Autodesk Inventor part; units mm, degrees
ref_plane "YZ Plane" through (0, 0, 0) normal (1, 0, 0) x (0, 1, 0)
ref_plane "XZ Plane" through (0, 0, 0) normal (0, 1, 0) x (-1, 0, 0)
ref_plane "XY Plane" through (0, 0, 0) normal (0, 0, 1) x (1, 0, 0)
sketch "Sketch2" plane through (0, 0, 0) normal (0, 1, 0) x (-1, 0, 0)
  circle A0 centre (0, 0) radius 10 construction
  circle A1 centre (0, 0) radius 9.9
  circle A2 centre (0, 0) radius 5 construction
  circle A3 centre (0, 0) radius 7 construction
  point P0 (0, 7)
  dimension "d8" = 14
  dimension "d5" = 20
  dimension "d6" = 0.1
  dimension "d7" = 10
extrude "Extrusion1" add sketch "Sketch2" along normal blind 3
sketch "Sketch3" plane through (0, 3, 0) normal (0, 1, 0) x (1, 0, 0)
  circle A0 centre (0, 0) radius 6.5 construction
  circle A1 centre (-6.5, 0) radius 0.75
  circle A2 centre (0, 0) radius 4
  circle A3 centre (0, 0) radius 8.5 construction
  circle A4 centre (0, -6.5) radius 2
  circle A5 centre (0, 6.5) radius 2
  circle A6 centre (-6.256, 1.7644) radius 0.75
  circle A7 centre (-5.5422, 3.3962) radius 0.75
  circle A8 centre (-4.4122, 4.7731) radius 0.75
  circle A9 centre (-2.9509, 5.7915) radius 0.75
  circle A10 centre (-6.256, -1.7644) radius 0.75
  circle A11 centre (-5.5422, -3.3962) radius 0.75
  circle A12 centre (-4.4122, -4.7731) radius 0.75
  circle A13 centre (-2.9509, -5.7915) radius 0.75
  circle A14 centre (-8.5, 0) radius 0.75
  circle A15 centre (-8.1604, -2.3785) radius 0.75
  circle A16 centre (-7.1688, -4.567) radius 0.75
  circle A17 centre (-5.6044, -6.3906) radius 0.75
  circle A18 centre (-3.5923, -7.7036) radius 0.75
  circle A19 centre (-8.1604, 2.3785) radius 0.75
  circle A20 centre (-7.1688, 4.567) radius 0.75
  circle A21 centre (-5.6044, 6.3906) radius 0.75
  circle A22 centre (-3.5923, 7.7036) radius 0.75
  circle A23 centre (0, 0) radius 9.9
  line L0 (0, -9.9) -> (0, 9.9) construction
  circle A24 centre (6.5, 0) radius 0.75
  circle A25 centre (6.256, 1.7644) radius 0.75
  circle A26 centre (5.5422, 3.3962) radius 0.75
  circle A27 centre (4.4122, 4.7731) radius 0.75
  circle A28 centre (2.9509, 5.7915) radius 0.75
  circle A29 centre (6.256, -1.7644) radius 0.75
  circle A30 centre (5.5422, -3.3962) radius 0.75
  circle A31 centre (4.4122, -4.7731) radius 0.75
  circle A32 centre (2.9509, -5.7915) radius 0.75
  arc A33 (3.5923, -7.7036) -> (8.5, 0) centre (0, 0) ccw construction
  circle A34 centre (3.5923, -7.7036) radius 0.35
  circle A35 centre (6.6057, -5.3492) radius 0.35
  circle A36 centre (8.2821, -1.9121) radius 0.35
  circle A37 centre (8.2821, 1.9121) radius 0.35
  circle A38 centre (6.6057, 5.3492) radius 0.35
  circle A39 centre (3.5923, 7.7036) radius 0.35
  dimension "d14" = 13
  dimension "d15" = 1.5
  dimension "d16" = 8
  dimension "d17" = 17
  dimension "d18" = 4
  dimension "d19" = 4
  dimension "d22" = 63
  dimension "d26" = 63
  dimension "d28" = 1.5
  dimension "d31" = 65
  dimension "d35" = 65
  dimension "d37" = 0.7
  dimension "d40" = 130
extrude "Extrusion2" cut sketch "Sketch3" against normal blind 3 contours A1 | A2 | A4 | A5 | A6 | A7 | A8 | A9 | A10 | A11 | A12 | A13 | A14 | A15 | A16 | A17 | A18 | A19 | A20 | A21 | A22 | A24 | A25 | A26 | A27 | A28 | A29 | A30 | A31 | A32 | A34 | A35 | A36 | A37 | A38 | A39
properties part number "top_housing_wire_guide"
The listing builds one solid part. Answer for the finished solid, in the listing's coordinates (mm). Round coordinates to 2 decimals unless told otherwise and drop trailing zeros. Loops run counter-clockwise (first coordinate to the right, second up) from the corner with the lowest first, then second, coordinate; pieces in that order, holes last. Notation, with made-up numbers: (-26.5, -7) -> (0.5, -7) arc R23 cw to (0.5, 30) -> close; hole circle Ø6 at (11.25, 54.5). An arc over 180 degrees is marked (long way). Use one line per item in the form item = value.
1. Find the intervals of material crossed by probe 1 along Z at (x, y) = (3, 1.85); probe 2 along Z at (x, y) = (-4.25, 0.4); probe 3 along X at (y, z) = (2.05, 6.75), in increasing order. Write a range as [from, to].
Answer key:
probe_1 = [-9.43, -6.54], [-5.04, -2.65], [2.65, 5.04], [6.54, 9.43]
probe_2 = [-8.94, -8.06], [-7.34, -5.51], [-4.04, 4.04], [5.51, 7.34], [8.06, 8.94]
probe_3 = [-7.24, -6.26], [-4.95, -1.98], [1.98, 7.24]
2. For a pull along Z with two mould halves and no side action, classify faces 1 (the cylindrical face through (3.817, 1.521, -4.317)), 2 (the cylindrical face through (-9.443, 1.479, -2.974)), 3 (the cylindrical face through (-3.72, 1.52, 5.06)) as released by +Z, released by -Z, zero draft, split by the parting line, or undercut.
Answer key:
face_1 = undercut
face_2 = split by the parting line
face_3 = undercut
3. The part is cut by section D-D on y = 2.15. Give the number of separate pieces and of enclosed holes in the cut face, and give its area (3 significant figures).
Answer key:
separate_pieces = 1
enclosed_holes = 36
area = 182 mm²
4. A flat-ended cylindrical pin translates along its axis: pin 1 Ø1.5 at (y, z) = (2.5, -7.5) entering from +X. Find the tip coordinate at first contact, or state that the pin passes through.
Answer key:
pin_1 = 7.24
5. The part is cut by section C-C on x = -8.5. Determine the outline of the cut face in (y, z).
Answer key:
outline = (0, -5.08) -> (3, -5.08) -> (3, -3.05) -> (0, -3.05) -> close; (0, -1.71) -> (3, -1.71) -> (3, -0.75) -> (0, -0.75) -> close; (0, 0.75) -> (3, 0.75) -> (3, 1.71) -> (0, 1.71) -> close; (0, 3.05) -> (3, 3.05) -> (3, 5.08) -> (0, 5.08) -> close
6. The part is cut by section B-B on z = -0.25. Determine the outline of the cut face in (x, y).
Answer key:
outline = (-9.9, 0) -> (-9.21, 0) -> (-9.21, 3) -> (-9.9, 3) -> close; (-7.79, 0) -> (-7.21, 0) -> (-7.21, 3) -> (-7.79, 3) -> close; (-5.79, 0) -> (-3.99, 0) -> (-3.99, 3) -> (-5.79, 3) -> close; (3.99, 0) -> (5.79, 0) -> (5.79, 3) -> (3.99, 3) -> close; (7.21, 0) -> (9.9, 0) -> (9.9, 3) -> (7.21, 3) -> close
7. The part is cut by section A-A on x = 0. Determine the outline of the cut face in (y, z), and give its area (3 significant figures).
Answer key:
outline = (0, -9.9) -> (3, -9.9) -> (3, -8.5) -> (0, -8.5) -> close; (0, -4.5) -> (3, -4.5) -> (3, -4) -> (0, -4) -> close; (0, 4) -> (3, 4) -> (3, 4.5) -> (0, 4.5) -> close; (0, 8.5) -> (3, 8.5) -> (3, 9.9) -> (0, 9.9) -> close
area = 11.4 mm²
